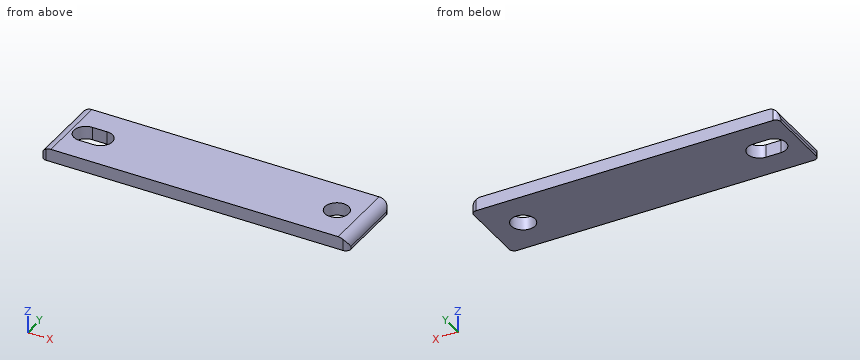
Autodesk Fusion 360 part; units mm, degrees
sketch "Sketch1" plane through (0, 0, 0) normal (0, 0, 1) x (1, 0, 0)
  line L0 (-31, 7.4) -> (31, 7.4)
  line L1 (31, 7.4) -> (31, -7.4)
  line L2 (31, -7.4) -> (-31, -7.4)
  line L3 (-31, -7.4) -> (-31, 7.4)
  line L4 (-31, 0) -> (31, 0) construction
  circle A0 centre (24.6, 0) radius 2.4
  line L5 (0, 7.4) -> (0, -7.4) construction
  circle A1 centre (-24.6, 0) radius 2.4 construction
  line L6 (-26.1, -2.4) -> (-23.1, -2.4)
  arc A2 (-23.1, -2.4) -> (-23.1, 2.4) centre (-23.1, 0) ccw
  line L7 (-23.1, 2.4) -> (-26.1, 2.4)
  arc A3 (-26.1, 2.4) -> (-26.1, -2.4) centre (-26.1, 0) ccw
  line L8 (-26.1, 0) -> (-23.1, 0) construction
  point P0 (-24.6, 0)
  dimension "d1" = 62
  dimension "d2" = 14.8
  dimension "d3" = 4.8
  dimension "d4" = 49.2
  dimension "d5" = 3
extrude "Extrude1" add sketch "Sketch1" along normal blind 2.6
fillet "Fillet2" radius 1 4 edges at (31, -7.4, 1.3) (31, 7.4, 1.3) (-31, 7.4, 1.3) (-31, -7.4, 1.3)
fillet "Fillet2" radius 2 2 edges at (31, 0, 2.6) (-31, 0, 2.6)
Could you check a few things on this model? Use its own coordinates, in mm. Give positions to 0.01 mm unless a question says otherwise; leave off trailing zeros. Order: outer loops, then holes, each group sorted by start corner. A loop starts at its lowest first (then second) coordinate and runs counter-clockwise, first axis right, second up. Notation, with made-up numbers: (60.5, -20) -> (117.5, -20) arc R6 ccw to (117.5, -12) -> close; hole circle Ø2 at (-11.5, 69). An arc over 180 degrees is marked (long way). Answer in a Markdown table with one row per item. Add a question column.
Item 1: Imagine slicing it at A-A (x = 24.6). List the corners of the cut face in (y, z) for me.
Item 2: Imagine slicing it at B-B (y = -1.5). List the corners of the cut face in (x, z) for me, and give its area (3 significant figures).
Item 3: Imagine slicing it at C-C (z = 1.1). List the corners of the cut face in (x, y) for me.
Item 4: Please list where these lines run through material, in increasing order: probe 1 along Y at (x, z) = (24.6, 1.4); probe 2 along X at (y, z) = (6.5, 0.65); probe 3 along Y at (x, z) = (23.5, 0.45).
Item 5: I'm going to push a flat-ended pin straight in: P1, Ø1, axis at y = 0.5, z = 1.5, coming from the +X side. Where does the tip first touch, or does it pass through?
Result:
| question | item | result |
|---|---|---|
| 1 | outline | (-7.4, 0) -> (-2.4, 0) -> (-2.4, 2.6) -> (-7.4, 2.6) -> close; (2.4, 0) -> (7.4, 0) -> (7.4, 2.6) -> (2.4, 2.6) -> close |
| 2 | outline | (-31, 0) -> (-27.97, 0) -> (-27.97, 2.6) -> (-29, 2.6) arc R2 ccw to (-31, 0.6) -> close; (-21.23, 0) -> (22.73, 0) -> (22.73, 2.6) -> (-21.23, 2.6) -> close; (26.47, 0) -> (31, 0) -> (31, 0.6) arc R2 ccw to (29, 2.6) -> (26.47, 2.6) -> close |
| 2 | area | 132 mm2 |
| 3 | outline | (-30.94, -6.75) arc R1 ccw to (-30, -7.4) -> (30, -7.4) arc R1 ccw to (30.94, -6.75) -> (30.94, 6.75) arc R1 ccw to (30, 7.4) -> (-30, 7.4) arc R1 ccw to (-30.94, 6.75) -> close; hole (-26.1, -2.4) -> (-23.1, -2.4) arc R2.4 ccw to (-23.1, 2.4) -> (-26.1, 2.4) arc R2.4 ccw to start; hole circle Ø4.8 at (24.6, 0) |
| 4 | probe 1 | -7.4 to -2.4, 2.4 to 7.4 |
| 4 | probe 2 | -30.99 to 30.99 |
| 4 | probe 3 | -7.4 to -2.13, 2.13 to 7.4 |
| 5 | P1 | x = 30.96 |
